Job drawing, mm, ordinate dimensions from the low corner. One solid piece. Coordinates: 2 decimals unless noted, no trailing zeros. Write each loop counter-clockwise with the first axis right and the second up, starting at its lowest first coordinate (ties: lowest second). Pieces come first, ordered by that corner, then holes. Notation, with made-up numbers: (10.25, 21.25) - (16.25, 21.25) arc R22 ccw to (16.25, 51.25) - close; hole circle Ø7 at (14, 89). An arc over 180 degrees is marked (long way). Put each result on its own line as item: value. Start each with the question number.
1. Drill centre lines: L1, parallel to X at y = 14.5, z = 2.95; L2, parallel to X at y = 23.5, z = 4.5. Where is each one in solid material? Low to high. Write a range as from..to.
2. Saw through at C-C, the plane y = 32. Write the cut outline in (x, z).
3. Saw through at A-A, the plane z = 4.15. Write the cut outline in (x, y).
4. Drop flat-ended pins along their axis: P1, Ø1.5, axis at y = 25, z = 2.5, coming from the +X side; P2, Ø3.5, axis at x = 157.09, y = 17.5, coming from the +Z side. Give the stop position or say it passes through.
5. Saw through at B-B, the plane y = 8. Write the cut outline in (x, z) (3 decimals), plus the area to 3 significant figures.
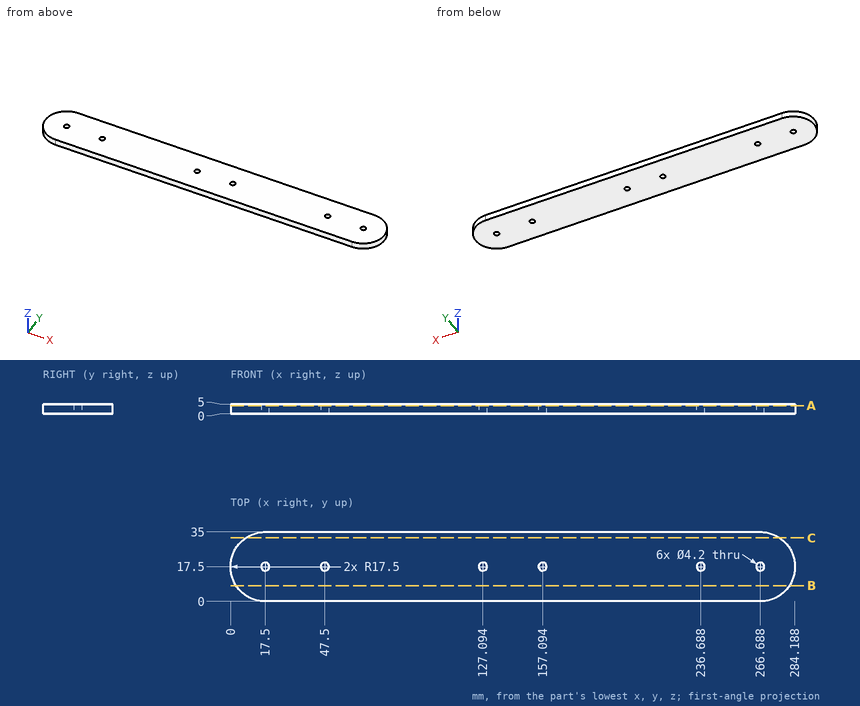
Final values:
1. L1: x = 0.26..283.93
1. L2: x = 1.06..283.13
2. outline: (7.7, 0) - (276.49, 0) - (276.49, 5) - (7.7, 5) - close
3. outline: (17.5, 0) - (266.69, 0) arc R17.5 ccw to (266.69, 35) - (17.5, 35) arc R17.5 ccw to start; hole circle Ø4.2 at (17.5, 17.5); hole circle Ø4.2 at (47.5, 17.5); hole circle Ø4.2 at (127.09, 17.5); hole circle Ø4.2 at (157.09, 17.5); hole circle Ø4.2 at (236.69, 17.5); hole circle Ø4.2 at (266.69, 17.5)
4. P1: stops at x = 282.83
4. P2: passes through
5. outline: (2.803, 0) - (281.385, 0) - (281.385, 5) - (2.803, 5) - close
5. area: 1,390 mm²
